Here's the drawing with two shaded views (mm, measured from the low corner). I have some questions. Give positions to 0.01 mm unless a question says otherwise; leave off trailing zeros. Loops run counter-clockwise (first coordinate to the right, second up) from the corner with the lowest first, then second, coordinate; pieces in that order, holes last. Notation, with made-up numbers: (-32.75, -8.75) - (0.25, -8.75) arc R17 ccw to (0.25, 19.25) - close; hole circle Ø2 at (42, 52.25). An arc over 180 degrees is marked (long way). Answer as a JSON object with one key per item and string values. Group by question number.
Item 1: Suppose I cut it at A-A on y = 104.5. Write out the boundary of the cut face in (x, z), and give its area (3 significant figures).
Item 2: Will this pin go through, and if not, where does the flat tip stop? pin 1 (1.5 mm diameter, centred on x = 103.5, y = 77.5, fed in from -Z).
Item 3: Suppose I cut it at C-C on z = 4.5. Write out the boundary of the cut face in (x, y), and give its area (3 significant figures).
Item 4: Please list where these lines run through material, in increasing order: L1, parallel to X at y = 104.5, z = 4; L2, parallel to Y at x = 19, z = 2.75.
Item 5: Suppose I cut it at D-D on y = 68. Write out the boundary of the cut face in (x, z), and give its area (3 significant figures).
Item 6: Thinking about a two-plate mould opening in X: for the marked faces 1, 2 and 3, which applies, pulls with the +X half, pulls with the -X half, needs draft (parallel to the pull), parting line crosses it, or undercut?
Item 7: Suppose I cut it at B-B on x = 12.5. Write out the boundary of the cut face in (y, z).
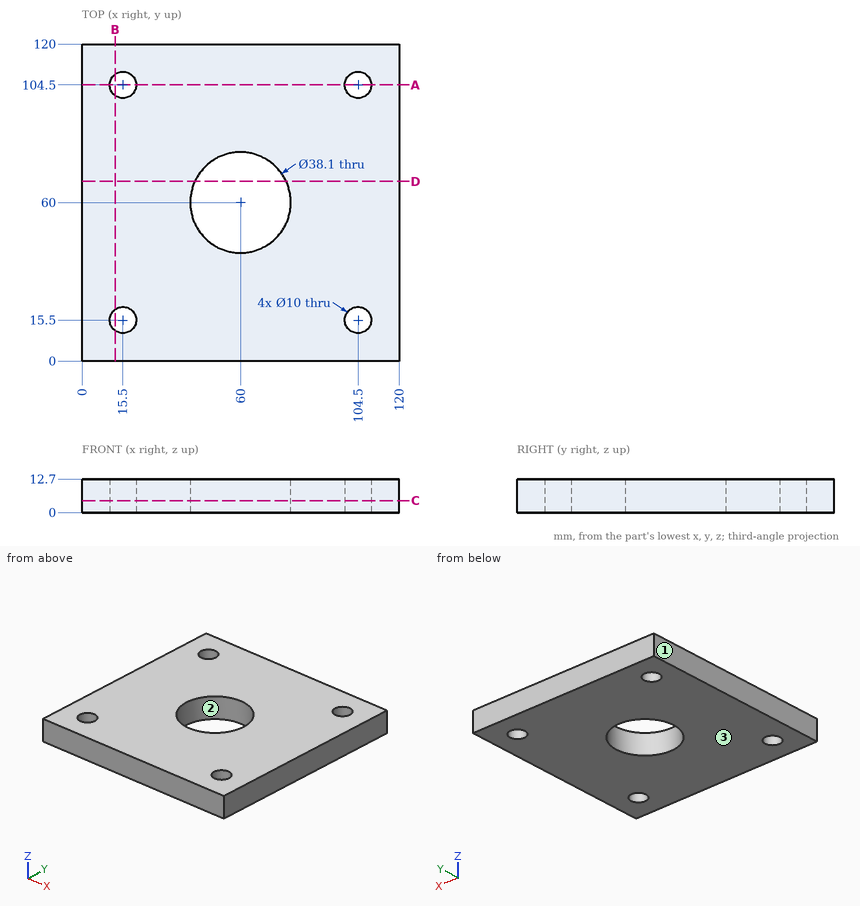
Worked out:
{
 "1": {"outline": "(0, 0) - (10.5, 0) - (10.5, 12.7) - (0, 12.7) - close; (20.5, 0) - (99.5, 0) - (99.5, 12.7) - (20.5, 12.7) - close; (109.5, 0) - (120, 0) - (120, 12.7) - (109.5, 12.7) - close", "area": "1,270 mm2"},
 "2": {"pin 1": "stops at z = 0"},
 "3": {"outline": "(0, 0) - (120, 0) - (120, 120) - (0, 120) - close; hole circle Ø10 at (15.5, 15.5); hole circle Ø10 at (15.5, 104.5); hole circle Ø38.1 at (60, 60); hole circle Ø10 at (104.5, 15.5); hole circle Ø10 at (104.5, 104.5)", "area": "12,900 mm2"},
 "4": {"L1": "x = 0 to 10.5, 20.5 to 99.5, 109.5 to 120", "L2": "y = 0 to 11.93, 19.07 to 100.93, 108.07 to 120"},
 "5": {"outline": "(0, 0) - (42.71, 0) - (42.71, 12.7) - (0, 12.7) - close; (77.29, 0) - (120, 0) - (120, 12.7) - (77.29, 12.7) - close", "area": "1,080 mm2"},
 "6": {"face 1": "pulls with the -X half", "face 2": "undercut", "face 3": "needs draft"},
 "7": {"outline": "(0, 0) - (11.5, 0) - (11.5, 12.7) - (0, 12.7) - close; (19.5, 0) - (100.5, 0) - (100.5, 12.7) - (19.5, 12.7) - close; (108.5, 0) - (120, 0) - (120, 12.7) - (108.5, 12.7) - close"}
}
